Can you work these out from the model? Positions are in its coordinate system, mm. Face numbers are marked on the shaded views. A direction names the side the tool comes from. Give positions to 0.01 mm unless a question says otherwise; leave off trailing zeros. Order: outer loops, then holes, each group sorted by start corner. A loop starts at its lowest first (then second) coordinate and runs counter-clockwise, first axis right, second up. Notation, with made-up numbers: (15.5, -8.5) - (40.5, -8.5) arc R28 ccw to (40.5, 16.5) - close; hole circle Ø6 at (-5.5, 18.25). An arc over 180 degrees is marked (long way). Use one line per item in the form item = value. Start each with the question number.
1) Suppose I cut it at B-B, the plane y = 6.75. Write out the boundary of the cut face in (x, z), and give its area (3 significant figures).
2) Suppose I cut it at C-C, the plane z = -26.5. Write out the boundary of the cut face in (x, y) (3 decimals).
3) Suppose I cut it at A-A, the plane x = 0. Write out the boundary of the cut face in (y, z) (3 decimals).
4) We'd pull the mould along Z, two halves only. Please class the marked faces 6, 7 and 8: released by +Z, released by -Z, zero draft, split by the parting line, or undercut.
5) Please list where these lines run through material, in increasing order: probe 1 along X at (y, z) = (6.75, -16.51); probe 2 along X at (y, z) = (11.95, 0); probe 3 along Z at (x, y) = (29, 10.5).
6) For pin 1 (12.5 mm diameter, centred on y = 8.5, z = -16.5, fed in from +X); pin 2 (5 mm diameter, centred on x = -8, y = 7.5, fed in from -Z); pin 3 (12.5 mm diameter, centred on x = -16.5, y = 9.5, fed in from +Z); pin 4 (5 mm diameter, centred on x = -18, z = 39, fed in from -Y), each with a flat end and sliding along its axis, tell me the tip position at first contact or that it passes through.
7) Which directions (+Z, -Z, +X, -X, +Y, -Y) give clear straight access to the entire face, cutting with the end or side of a thin tool? Please do the marked faces 1, 2, 3, 4 and 5.
8) Suppose I cut it at D-D, the plane z = -16.51. Write out the boundary of the cut face in (x, y) (3 decimals).
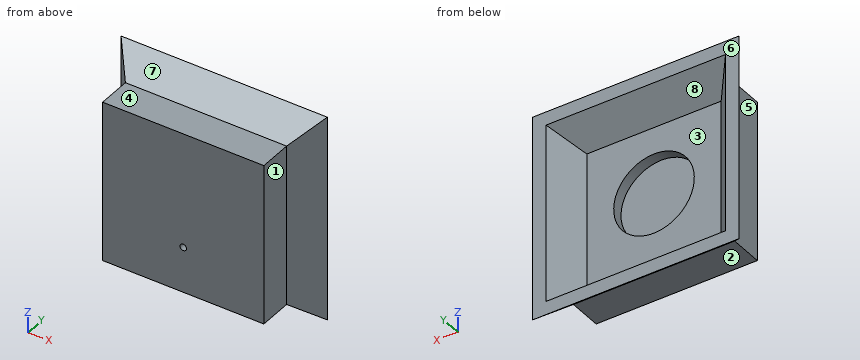
```python
from build123d import *

# Parameters (mm, degrees)
SKETCH1_W               = 76.2
SKETCH1_H               = 76.2
BOSS_EXTRUDE1_DEPTH     = 15.875
SKETCH2_W               = 76.2
SKETCH2_H               = 76.2
BOSS_EXTRUDE2_DEPTH     = 12.7
BOSS_EXTRUDE2_DRAFT     = -40
MIRROR1_COPY_1_SKETCH_W = 76.2
MIRROR1_COPY_1_SKETCH_H = 76.2
MIRROR1_COPY_1_DEPTH    = 12.7
MIRROR1_COPY_1_DRAFT    = -40
SKETCH4_W               = 84.813130632
SKETCH4_H               = 84.813130632
CUT_EXTRUDE2_DEPTH      = 12.7
CUT_EXTRUDE2_DRAFT      = -40
SKETCH5_R               = 19.05
CUT_EXTRUDE3_DEPTH      = 5.08
SKETCH6_R               = 1.524
CUT_EXTRUDE4_DEPTH      = 20.32
CUT_EXTRUDE5_REACH      = 76.639
SKETCH8_W               = 110.353971767
SKETCH8_H               = 106.914185114


with BuildPart() as part:
    # Sketch1 → Boss-Extrude1 (new, symmetric)
    with BuildSketch(Plane(origin=(0, 0, 0), x_dir=(1, 0, 0), z_dir=(0, 1, 0))):
        Rectangle(SKETCH1_W, SKETCH1_H)
    extrude(amount=BOSS_EXTRUDE1_DEPTH, both=True)


with BuildPart() as boss_extrude2_tool:
    # Sketch2 → Boss-Extrude2 (with draft: the straight prism first)
    with BuildSketch(Plane(origin=(0, 15.875, 0), x_dir=(1, 0, 0), z_dir=(0, 1, 0))):
        Rectangle(SKETCH2_W, SKETCH2_H)
    extrude(amount=BOSS_EXTRUDE2_DEPTH)
    # Boss-Extrude2: the draft: its side faces are tilted about the plane it starts from
    boss_extrude2_sides = [boss_extrude2_tool.faces().sort_by_distance(p)[0] for p in [
        (-38.1, 22.225, 0),
        (0, 22.225, 38.1),
        (38.1, 22.225, 0),
        (0, 22.225, -38.1),
    ]]
    draft(boss_extrude2_sides, Plane(origin=(0, 15.875, 0), x_dir=(1, 0, 0), z_dir=(0, 1, 0)), BOSS_EXTRUDE2_DRAFT)


with BuildPart() as part_1:
    add(part.part)

    # Boss-Extrude2: add boss_extrude2_tool
    add(boss_extrude2_tool.part)


with BuildPart() as mirror1_copy_1_tool:
    # Mirror1 copy 1 sketch → Mirror1 copy 1 (with draft: the straight prism first)
    with BuildSketch(Plane.XZ.offset(15.875)):
        Rectangle(MIRROR1_COPY_1_SKETCH_W, MIRROR1_COPY_1_SKETCH_H)
    extrude(amount=MIRROR1_COPY_1_DEPTH)
    # Mirror1 copy 1: the draft: its side faces are tilted about the plane it starts from
    mirror1_copy_1_sides = [mirror1_copy_1_tool.faces().sort_by_distance(p)[0] for p in [
        (-38.1, -22.225, 0),
        (0, -22.225, 38.1),
        (38.1, -22.225, 0),
        (0, -22.225, -38.1),
    ]]
    draft(mirror1_copy_1_sides, Plane.XZ.offset(15.875), MIRROR1_COPY_1_DRAFT)


with BuildPart() as part_2:
    add(part_1.part)

    # Mirror1 copy 1: add mirror1_copy_1_tool
    add(mirror1_copy_1_tool.part)


with BuildPart() as cut_extrude2_tool:
    # Sketch4 → Cut-Extrude2 (with draft: the straight prism first)
    with BuildSketch(Plane(origin=(0, 28.575, 0), x_dir=(1, 0, 0), z_dir=(0, 1, 0))):
        Rectangle(SKETCH4_W, SKETCH4_H)
    extrude(amount=-CUT_EXTRUDE2_DEPTH)
    # Cut-Extrude2: the draft: its side faces are tilted about the plane it starts from
    cut_extrude2_sides = [cut_extrude2_tool.faces().sort_by_distance(p)[0] for p in [
        (42.406565316, 22.225, 0),
        (0, 22.225, -42.406565316),
        (-42.406565316, 22.225, 0),
        (0, 22.225, 42.406565316),
    ]]
    draft(cut_extrude2_sides, Plane(origin=(0, 28.575, 0), x_dir=(1, 0, 0), z_dir=(0, 1, 0)), CUT_EXTRUDE2_DRAFT)


with BuildPart() as part_3:
    add(part_2.part)

    # Cut-Extrude2: cut by cut_extrude2_tool
    add(cut_extrude2_tool.part, mode=Mode.SUBTRACT)

    # Sketch5 → Cut-Extrude3 (cut)
    with BuildSketch(Plane(origin=(0, 15.875, 0), x_dir=(1, 0, 0), z_dir=(0, 1, 0))):
        with Locations(Location((0, 0, 0), (0, 0, 270))):
            Circle(SKETCH5_R)
    extrude(amount=-CUT_EXTRUDE3_DEPTH, mode=Mode.SUBTRACT)

    # Sketch6 → Cut-Extrude4 (cut)
    with BuildSketch(Plane(origin=(0, 10.795, 0), x_dir=(1, 0, 0), z_dir=(0, 1, 0))):
        with Locations(Location((0, 16.51, 0), (0, 0, 270))):
            Circle(SKETCH6_R)
    extrude(amount=-CUT_EXTRUDE4_DEPTH, mode=Mode.SUBTRACT)

    # Sketch8 → Cut-Extrude5 (cut, up to next)
    with BuildSketch(Plane(origin=(0, 0, 0), x_dir=(1, 0, 0), z_dir=(0, 1, 0)), mode=Mode.PRIVATE) as cut_extrude5_sk1:
        with Locations((3.158987741, -3.05368815)):
            Rectangle(SKETCH8_W, SKETCH8_H)
    cut_extrude5_tool1 = extrude(cut_extrude5_sk1.sketch, amount=-CUT_EXTRUDE5_REACH, mode=Mode.PRIVATE) & part_3.part
    add(cut_extrude5_tool1.solids().sort_by_distance((3.158988, 0, 3.053688))[0], mode=Mode.SUBTRACT)


solid = part_3.part
```
Result sheet:
q1.outline = (-38.1, -38.1) - (38.1, -38.1) - (38.1, 38.1) - (-38.1, 38.1) - close; hole circle Ø3.05 at (0, -16.51)
q1.area = 5,800 mm²
q2.outline = (-48.757, 28.575) - (-38.1, 15.875) - (-38.1, 0) - (38.1, 0) - (38.1, 15.875) - (48.757, 28.575) - (42.407, 28.575) - (31.75, 15.875) - (-31.75, 15.875) - (-42.407, 28.575) - close
q3.outline = (0, -38.1) - (15.875, -38.1) - (28.575, -48.757) - (28.575, -42.407) - (15.875, -31.75) - (15.875, -19.05) - (10.795, -19.05) - (10.795, -18.034) - (0, -18.034) - close; (0, -14.986) - (10.795, -14.986) - (10.795, 19.05) - (15.875, 19.05) - (15.875, 31.75) - (28.575, 42.407) - (28.575, 48.757) - (15.875, 38.1) - (0, 38.1) - close
q4.face_6 = zero draft
q4.face_7 = released by +Z
q4.face_8 = undercut
q5.probe_1 = -38.1 to -1.52, 1.52 to 38.1
q5.probe_2 = -38.1 to -19.05, 19.05 to 38.1
q5.probe_3 = -38.1 to 38.1
q6.pin_1 = 38.1
q6.pin_2 = -38.1
q6.pin_3 = 38.1
q6.pin_4 = 0
q7.face_1 = +Z, -Z, +X, -Y
q7.face_2 = -Z, +X, -X, -Y
q7.face_3 = +Y
q7.face_4 = +Z, +X, -X, -Y
q7.face_5 = +Z, -Z, -X, -Y
q8.outline = (-48.757, 28.575) - (-38.1, 15.875) - (-38.1, 0) - (-1.524, 0) - (-1.524, 10.795) - (-9.504, 10.795) - (-9.504, 15.875) - (-31.75, 15.875) - (-42.407, 28.575) - close; (1.524, 0) - (38.1, 0) - (38.1, 15.875) - (48.757, 28.575) - (42.407, 28.575) - (31.75, 15.875) - (9.504, 15.875) - (9.504, 10.795) - (1.524, 10.795) - close
